```python
from build123d import *

# Parameters (mm, degrees)
CUT_EXTRUDE_1_DEPTH = 1.15
FILLET_1_R          = 0.4
FILLET_2_R          = 0.8


with BuildPart() as part:
    # 草圖1 → 旋轉1 (revolve)
    with BuildSketch(Plane.XY, mode=Mode.PRIVATE) as revolve_1_sk:
        Polygon((-2.3, 4), (-2.3, 0), (7.7, 0), (7.7, 2), (1.4, 2), (0.7, 1.78525), (0.21475, 1.78525), (-2, 4), align=None)
    revolve(revolve_1_sk.sketch.rotate(Axis((-2.3, 0, 0), (1, 0, 0)), 270), axis=Axis((-2.3, 0, 0), (1, 0, 0)))

    # 草圖2 → 除料-伸長1 (cut)
    with BuildSketch(Plane.ZY.offset(2.3)):
        Polygon((0.533333333, -0.533333333), (2.25, -0.533333333), (2.25, 0.533333333), (0.533333333, 0.533333333), (0.533333333, 2.25), (-0.533333333, 2.25), (-0.533333333, 0.533333333), (-2.25, 0.533333333), (-2.25, -0.533333333), (-0.533333333, -0.533333333), (-0.533333333, -2.25), (0.533333333, -2.25), align=None)
    extrude(amount=-CUT_EXTRUDE_1_DEPTH, mode=Mode.SUBTRACT)

    # 圓角1
    fillet_1_edges = [part.edges().sort_by_distance(p)[0] for p in [
        (0.21475, 0, 1.78525),
    ]]
    fillet(fillet_1_edges, radius=FILLET_1_R)

    # 圓角2
    fillet_2_edges = [part.edges().sort_by_distance(p)[0] for p in [
        (-1.725, -0.533333333, 0.533333333),
        (-1.725, -0.533333333, -0.533333333),
        (-1.725, 0.533333333, -0.533333333),
        (-1.725, 0.533333333, 0.533333333),
    ]]
    fillet(fillet_2_edges, radius=FILLET_2_R)


solid = part.part
```
Build history of the part. All positions in model axes, mm. A direction names the side the tool comes from. Round coordinates to 2 decimals unless told otherwise and drop trailing zeros. Write each loop counter-clockwise with the first axis right and the second up, starting at its lowest first coordinate (ties: lowest second). Pieces come first, ordered by that corner, then holes. Notation, with made-up numbers: (38.5, 19) - (50.5, 19) arc R22 ccw to (50.5, 27) - close; hole circle Ø8 at (34.25, 33). An arc over 180 degrees is marked (long way). Write each question's results on one line, items separated by ' | '. Start each with the question number.
Item 1: Which spindle directions (+Z, -Z, +X, -X, +Y, -Y) get a long thin tool onto all of the face, cutting with end or side? Do faces 1 (the face through (0.54, -0.68, -1.65)), 2 (the face through (5, -2, 0)), 3 (the face through (-2, -0.533, -2)). Say none if no direction does.
Item 2: Saw through at A-A (x = 4.75). Write the cut outline in (y, z).
Item 3: Mould opens along Y. For faces 4 (the face through (-0.034, -0.779, -1.879)), 5 (the face through (-2, 0, 2.25)), 6 (the face through (-2.3, -1, -1)) say: pulls with the +Y half, pulls with the -Y half, needs draft (parallel to the pull), parting line crosses it, or undercut.
Item 4: Wall check: L1, parallel to X at y = -0.5, z = -1; L2, parallel to X at y = 3, z = 2.5; L3, parallel to Z at x = -1.25, y = 2. Give the ranges that are in metal, low to high. Write a range as [from, to].
Item 5: Drop flat-ended pins along their axis: P1, Ø2, axis at x = 2.5, z = -1.5, coming from the -Y side; P2, Ø0.5, axis at x = -1.5, y = -1.5, coming from the +Z side; P3, Ø4, axis at x = 5.5, z = -3, coming from the +Y side. Give the stop position or say it passes through.
Results are:
1) face 1: none | face 2: +X | face 3: -X
2) outline: circle Ø4 at (0, 0)
3) face 4: parting line crosses it | face 5: undercut | face 6: needs draft
4) L1: x = [-1.15, 7.7] | L2: x = [-2.3, -1.91] | L3: z = [-2.56, -0.53], [0.53, 2.56]
5) P1: stops at y = -1.94 | P2: stops at z = 3.46 | P3: stops at y = 1.73
